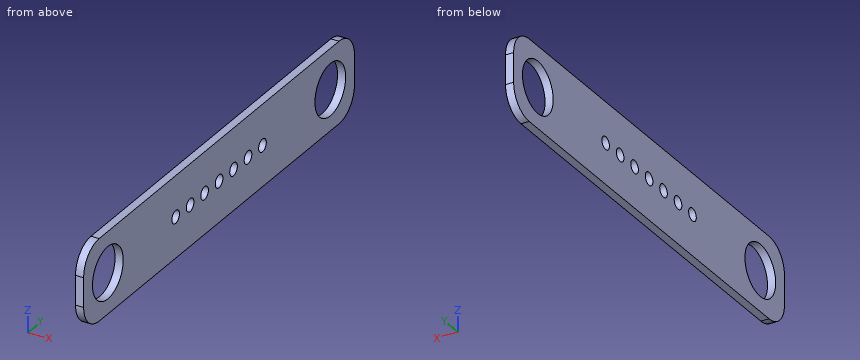
```python
from build123d import *

# Parameters (mm, degrees)
SKETCH1_W               = 88.9
SKETCH1_H               = 15.875
BASE_FLANGE1_DEPTH      = 1.5875
F_2_5MM_DOWEL_HOLE1_D   = 2.5
LPATTERN1_COUNT         = 4
LPATTERN1_PITCH         = 4.750000025
LPATTERN1_COL_COUNT     = 4
LPATTERN1_COL_PITCH     = 4.750000025
FILLET1_R               = 5.08
F_3_8_CLEARANCE_HOLE1_D = 10.0838


# Sheet-metal steps are written as plain solids
with BuildPart() as part:
    # Sketch1 → Base-Flange1 (new body)
    with BuildSketch(Plane.YZ):
        Rectangle(SKETCH1_W, SKETCH1_H)
    extrude(amount=-BASE_FLANGE1_DEPTH)

    # Ø2.5mm Dowel Hole1 (through all)
    with Locations(Plane(origin=(-1.5875, 0, 0), x_dir=(0, -1, 0), z_dir=(-1, 0, 0))):
        with Locations((0, 0)):
            f_2_5mm_dowel_hole1 = Hole(F_2_5MM_DOWEL_HOLE1_D / 2)

    # LPattern1: Ø2.5mm Dowel Hole1 ×4
    with Locations(*[(0, -i * LPATTERN1_PITCH, 0) for i in range(1, LPATTERN1_COUNT)]):
        add(f_2_5mm_dowel_hole1, mode=Mode.SUBTRACT)

    # LPattern1 col: Ø2.5mm Dowel Hole1 ×4
    with Locations(*[(0, i * LPATTERN1_COL_PITCH, 0) for i in range(1, LPATTERN1_COL_COUNT)]):
        add(f_2_5mm_dowel_hole1, mode=Mode.SUBTRACT)

    # Fillet1
    fillet1_edges = [part.edges().sort_by_distance(p)[0] for p in [
        (-0.79375, -44.45, 7.9375),
        (-0.79375, 44.45, 7.9375),
        (-0.79375, 44.45, -7.9375),
        (-0.79375, -44.45, -7.9375),
    ]]
    fillet(fillet1_edges, radius=FILLET1_R)

    # 3/8 Clearance Hole1 (through all)
    with Locations(Plane(origin=(-1.5875, 0, 0), x_dir=(0, -1, 0), z_dir=(-1, 0, 0))):
        with Locations((-36.5125, 0), (36.5125, 0)):
            Hole(F_3_8_CLEARANCE_HOLE1_D / 2)


solid = part.part
```
The listing builds one solid part. Answer for the finished solid, in the listing's coordinates (mm). Round coordinates to 2 decimals unless told otherwise and drop trailing zeros. Loops run counter-clockwise (first coordinate to the right, second up) from the corner with the lowest first, then second, coordinate; pieces in that order, holes last.
1) A cutting plane is placed at B-B on x = -0.45. Give the number of separate pieces and of enclosed holes in the cut face, plus the area to 3 significant figures.
Outcome:
separate pieces: 1
enclosed holes: 9
area: 1,200 mm2
2) A cutting plane is placed at D-D on z = 6. Determine the outline of the cut face in (x, y).
Outcome:
outline: (-1.59, -43.36) - (0, -43.36) - (0, 43.36) - (-1.59, 43.36) - close
3) A cutting plane is placed at A-A on y = -4.75. Determine the outline of the cut face in (x, z), plus the area to 3 significant figures.
Outcome:
outline: (-1.59, -7.94) - (0, -7.94) - (0, -1.25) - (-1.59, -1.25) - close; (-1.59, 1.25) - (0, 1.25) - (0, 7.94) - (-1.59, 7.94) - close
area: 21.2 mm2
4) Consider line 1 (Z direction, x = -0.9, y = -4.75); line 2 (Y direction, x = -1.5, z = -2.5); line 3 (Y direction, x = -1.15, z = -1.75). Determine where each line is inside the solid, lowest interval first.
Outcome:
line 1: z = -7.94 to -1.25, 1.25 to 7.94
line 2: y = -44.45 to -40.89, -32.13 to 32.13, 40.89 to 44.45
line 3: y = -44.45 to -41.24, -31.78 to 31.78, 41.24 to 44.45
5) Given P1, Ø9, axis at y = -36.51, z = 0, coming from the -X side, flat-ended and moving along its own axis, determine where the tip first touches the part or whether it passes through.
Outcome:
P1: passes through
6) A cutting plane is placed at C-C on z = 2. Determine the outline of the cut face in (x, y).
Outcome:
outline: (-1.59, -44.45) - (0, -44.45) - (0, -41.14) - (-1.59, -41.14) - close; (-1.59, -31.88) - (0, -31.88) - (0, 31.88) - (-1.59, 31.88) - close; (-1.59, 41.14) - (0, 41.14) - (0, 44.45) - (-1.59, 44.45) - close
